Check sheet for the modelled part. Datum: model origin and axes. Units: mm. Face numbers are marked on the shaded views. A direction names the side the tool comes from. Give positions to 0.01 mm unless a question says otherwise; leave off trailing zeros. Write each loop counter-clockwise with the first axis right and the second up, starting at its lowest first coordinate (ties: lowest second). Pieces come first, ordered by that corner, then holes. Notation, with made-up numbers: (82, 83) - (91, 83) arc R25 ccw to (91, 95) - close; hole circle Ø7 at (50.25, 79.25). An arc over 180 degrees is marked (long way). Return JSON: item names as keys, results as strings. Group by question number.
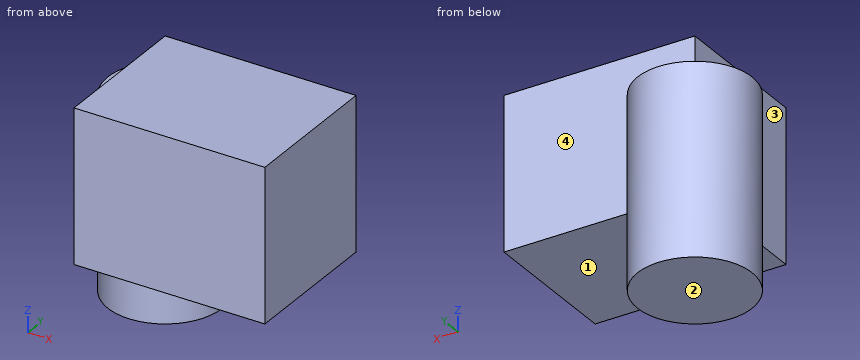
```python
from build123d import *

# Parameters (mm, degrees)
SKETCH_W     = 25
SKETCH_H     = 20
PAD_DEPTH    = 19
SKETCH001_R  = 7.5
PAD001_DEPTH = 12.5


with BuildPart() as part:
    # Sketch → Pad (new body)
    with BuildSketch(Plane.XZ):
        with Locations((12.5, 10)):
            Rectangle(SKETCH_W, SKETCH_H)
    extrude(amount=PAD_DEPTH)

    # Sketch001 → Pad001 (join, symmetric)
    with BuildSketch(Plane.XY):
        Circle(SKETCH001_R)
    extrude(amount=PAD001_DEPTH, both=True)


solid = part.part
```
Item 1: Access from +Z, -Z, +X, -X, +Y, -Y to the whole of each face (thin tool, end or side, straight path). Record for the marked faces 1, 2, 3 and 4.
Item 2: Section check C-C on y = -2. Record the cut outline in (x, z), plus the area to 3 significant figures.
Item 3: Material ranges on line 1 along Z through (x, y) = (-4, -5.5); line 2 along Y through (x, z) = (2, 17); line 3 along X through (y, z) = (-16, 0.5), recorded low to high. Write a range as from..to.
Item 4: Section check D-D on x = 10. Record the cut outline in (y, z), plus the area to 3 significant figures.
Item 5: Section check A-A on x = 6. Record the cut outline in (y, z), plus the area to 3 significant figures.
Item 6: Depth check by flat-ended pin: pin 1 (16 mm diameter, centred on x = 13.5, z = 10.5, fed in from +Y); pin 2 (1.5 mm diameter, centred on x = 2, z = -5, fed in from +Y); pin 3 (1.5 mm diameter, centred on x = 10.5, z = 0.5, fed in from +Y). Enter the tip coordinate at first touch or a pass-through.
Item 7: Section check B-B on z = 4. Record the cut outline in (x, y).
Reply:
{
 "1": {"face 1": "-Z, +X, -Y", "face 2": "-Z, +X, -X, +Y, -Y", "face 3": "+Z, -X, -Y", "face 4": "+Z, +X, +Y"},
 "2": {"outline": "(-7.23, -12.5) - (7.23, -12.5) - (7.23, 0) - (25, 0) - (25, 20) - (0, 20) - (0, 12.5) - (-7.23, 12.5) - close", "area": "771 mm²"},
 "3": {"line 1": "-12.5..12.5", "line 2": "-19..0", "line 3": "0..25"},
 "4": {"outline": "(-19, 0) - (0, 0) - (0, 20) - (-19, 20) - close", "area": "380 mm²"},
 "5": {"outline": "(-19, 0) - (-4.5, 0) - (-4.5, -12.5) - (4.5, -12.5) - (4.5, 12.5) - (0, 12.5) - (0, 20) - (-19, 20) - close", "area": "549 mm²"},
 "6": {"pin 1": "y = 5.1", "pin 2": "y = 7.4", "pin 3": "y = 0"},
 "7": {"outline": "(0, -19) - (25, -19) - (25, 0) - (7.5, 0) arc R7.5 ccw (long way) to (0, -7.5) - close"}
}
